The model under review builds one solid part; all positions refer to its coordinate system, in mm. A direction names the side the tool comes from. Round coordinates to 2 decimals unless told otherwise and drop trailing zeros. Write each loop counter-clockwise with the first axis right and the second up, starting at its lowest first coordinate (ties: lowest second). Pieces come first, ordered by that corner, then holes. Notation, with made-up numbers: (70, 23) - (96, 23) arc R14 cw to (96, 36) - close; hole circle Ø11 at (-40, 20.25). An arc over 180 degrees is marked (long way). Write each question's results on one line, items separated by ' | '.
```python
from build123d import *

# Parameters (mm, degrees)
SKETCH1_R           = 1.5
BOSS_EXTRUDE1_DEPTH = 1.5
FILLET1_R           = 2
SKETCH2_R           = 1
CUT_EXTRUDE1_DEPTH  = 5


with BuildPart() as part:
    # Sketch1 → Boss-Extrude1 (new body)
    with BuildSketch(Plane.XY):
        with BuildLine():
            Line((-5.5, -11.303847577), (-3, -11.303847577))
            ThreePointArc((-3, -11.303847577), (-4.5, -9.803847577), (-3, -8.303847577))
            Line((-3, -8.303847577), (-8.5, -8.303847577))
            Line((-8.5, -8.303847577), (-8.5, -108.303847577))
            Line((-8.5, -108.303847577), (-0.5, -108.303847577))
            Line((-0.5, -108.303847577), (-0.5, -68.303847577))
            Line((-0.5, -68.303847577), (-5.5, -63.303847577))
            Line((-5.5, -63.303847577), (-5.5, -51.696152423))
            Line((-5.5, -51.696152423), (-3, -51.696152423))
            ThreePointArc((-3, -51.696152423), (-4.5, -50.196152423), (-3, -48.696152423))
            Line((-3, -48.696152423), (-5.5, -48.696152423))
            Line((-5.5, -48.696152423), (-5.5, -41.303847577))
            Line((-5.5, -41.303847577), (-3, -41.303847577))
            ThreePointArc((-3, -41.303847577), (-4.5, -39.803847577), (-3, -38.303847577))
            Line((-3, -38.303847577), (-5.5, -38.303847577))
            Line((-5.5, -38.303847577), (-5.5, -21.696152423))
            Line((-5.5, -21.696152423), (-3, -21.696152423))
            ThreePointArc((-3, -21.696152423), (-4.5, -20.196152423), (-3, -18.696152423))
            Line((-3, -18.696152423), (-5.5, -18.696152423))
            Line((-5.5, -18.696152423), (-5.5, -11.303847577))
        make_face()
        with Locations((-3, -39.803847577)):
            Circle(SKETCH1_R)
        with Locations((-3, -50.196152423)):
            Circle(SKETCH1_R)
        with Locations((-3, -9.803847577)):
            Circle(SKETCH1_R)
        with Locations((-3, -20.196152423)):
            Circle(SKETCH1_R)
    extrude(amount=BOSS_EXTRUDE1_DEPTH)

    # Fillet1
    fillet1_edges = [part.edges().sort_by_distance(p)[0] for p in [
        (-5.5, -51.696152423, 0.75),
        (-5.5, -11.303847577, 0.75),
        (-5.5, -18.696152423, 0.75),
        (-5.5, -21.696152423, 0.75),
        (-5.5, -38.303847577, 0.75),
        (-5.5, -41.303847577, 0.75),
        (-5.5, -48.696152423, 0.75),
    ]]
    fillet(fillet1_edges, radius=FILLET1_R)

    # Sketch2 → Cut-Extrude1 (cut)
    with BuildSketch(Plane.XY.offset(1.5)):
        with Locations((-5.5, -104.303847577)):
            Circle(SKETCH2_R)
        with Locations((-5.5, -84.303847577)):
            Circle(SKETCH2_R)
    extrude(amount=-CUT_EXTRUDE1_DEPTH, mode=Mode.SUBTRACT)


solid = part.part
```
Q1. Insertion check: P1, Ø1.2, axis at x = -5.5, y = -104.3, coming from the -Z side; P2, Ø0.8, axis at y = -14.5, z = 0.5, coming from the +X side. Each pin has a flat end and moves straight along its axis. Give the tip position at first contact, or say it passes through.
Evaluation:
P1: passes through | P2: stops at x = -5.5
Q2. Tool access review of faces 5 (the flat face through (-5, -69, 1.5)), 6 (the cylindrical face through (-4.899, -48.126, 0.76)): name each direction out of +Z, -Z, +X, -X, +Y, -Y from which nothing blocks a thin tool from reaching the whole face with its end or side.
Evaluation:
face 5: +Z, +X, -X, +Y, -Y | face 6: +Z, -Z, +X
Q3. We need section A-A (z = 0.9). State how many separate pieces and enclosed holes the cut face has, plus the area to 3 significant figures.
Evaluation:
separate pieces: 1 | enclosed holes: 2 | area: 556 mm^2
Q4. We need section B-B (y = -15.5). State the section outline as (x, z) points.
Evaluation:
outline: (-8.5, 0) - (-5.5, 0) - (-5.5, 1.5) - (-8.5, 1.5) - close
Q5. The part is to be moulded in two halves that separate along X. For faces 1 (the cylindrical face through (-5.63, -103.312, 0.76)), 2 (the flat face through (-5, -69, 0)), 3 (the cylindrical face through (-5.63, -83.312, 0.76)), 4 (the cylindrical face through (-4.93, -52.3, 0.76)), say which applies: released by +X, released by -X, zero draft, split by the parting line, or undercut.
Evaluation:
face 1: undercut | face 2: zero draft | face 3: undercut | face 4: released by +X
Q6. For probe 1 along Y at (x, z) = (-5.75, 1.05); probe 2 along Y at (x, z) = (-6, 0.6); probe 3 along X at (y, z) = (-33.5, 0.65), list the stretches that pass through material, from the lowest coordinate up.
Evaluation:
probe 1: y = -108.3 to -105.27, -103.34 to -85.27, -83.34 to -8.3 | probe 2: y = -108.3 to -105.17, -103.44 to -85.17, -83.44 to -8.3 | probe 3: x = -8.5 to -5.5
